Part model, mm, in its own coordinate system. Face numbers are marked on the shaded views. Coordinates: 2 decimals unless noted, no trailing zeros. Write each loop counter-clockwise with the first axis right and the second up, starting at its lowest first coordinate (ties: lowest second). Pieces come first, ordered by that corner, then holes. Notation, with made-up numbers: (1.25, 29.25) - (20.25, 29.25) arc R20 cw to (20.25, 57.25) - close; hole circle Ø10 at (-20, 2). An arc over 180 degrees is marked (long way). Use a Markdown table: item, result.
```python
from build123d import *

# Parameters (mm, degrees)
STOCK_MULTIBODY_1_OUTLINE_R   = 1.6
STOCK_MULTIBODY_1_OUTLINE_R_2 = 8.85
STOCK_MULTIBODY_1_DEPTH       = 17.5
CUT_EXTRUDE1_DEPTH            = 33.06633749
CUT_EXTRUDE1_DEPTH_BACK       = 33.06633749
SKETCH1_R                     = 17.5


# Read off the part's stored shape, not the designer's step: Stock-Multibody-1
with BuildPart() as part:
    # Stock-Multibody-1 outline → Stock-Multibody-1 (new body)
    with BuildSketch(Plane(origin=(0, 0, 0), x_dir=(1, 0, 0), z_dir=(0, 1, 0))):
        with BuildLine():
            ThreePointArc((-19, -17), (-18.414213562, -18.414213562), (-17, -19))
            Line((-17, -19), (17, -19))
            ThreePointArc((17, -19), (18.414213562, -18.414213562), (19, -17))
            Line((19, -17), (19, 17))
            ThreePointArc((19, 17), (18.414213562, 18.414213562), (17, 19))
            Line((17, 19), (-17, 19))
            ThreePointArc((-17, 19), (-18.414213562, 18.414213562), (-19, 17))
            Line((-19, 17), (-19, -17))
        make_face()
        with Locations((-14.8, -14.8)):
            Circle(STOCK_MULTIBODY_1_OUTLINE_R, mode=Mode.SUBTRACT)
        with Locations((14.8, -14.8)):
            Circle(STOCK_MULTIBODY_1_OUTLINE_R, mode=Mode.SUBTRACT)
        with Locations((-14.8, 14.8)):
            Circle(STOCK_MULTIBODY_1_OUTLINE_R, mode=Mode.SUBTRACT)
        Circle(STOCK_MULTIBODY_1_OUTLINE_R_2, mode=Mode.SUBTRACT)
        with Locations((14.8, 14.8)):
            Circle(STOCK_MULTIBODY_1_OUTLINE_R, mode=Mode.SUBTRACT)
    extrude(amount=STOCK_MULTIBODY_1_DEPTH)

    # Sketch1 → Cut-Extrude1 (cut, two sides: drawn at the far end of the back side and taken through both)
    with BuildSketch(Plane(origin=(0, 17.5, 0), x_dir=(1, 0, 0), z_dir=(0, 1, 0)).offset(-CUT_EXTRUDE1_DEPTH_BACK)):
        with Locations(Location((0, 0, 0), (0, 0, 270))):
            Circle(SKETCH1_R)
    extrude(amount=CUT_EXTRUDE1_DEPTH + CUT_EXTRUDE1_DEPTH_BACK, mode=Mode.SUBTRACT)


solid = part.part
```
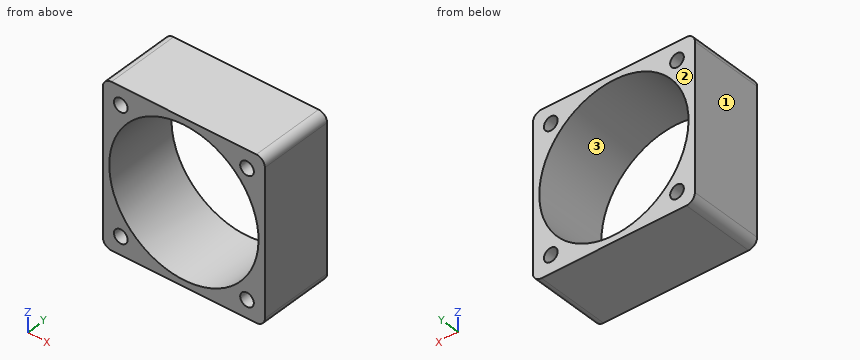
Item 1: Band-saw the part on C-C, the plane y = 9. Give the cut face in (x, z), then the cut area to 3 significant figures.
From the geometry:
| item | result |
|---|---|
| outline | (-19, -17) arc R2 ccw to (-17, -19) - (17, -19) arc R2 ccw to (19, -17) - (19, 17) arc R2 ccw to (17, 19) - (-17, 19) arc R2 ccw to (-19, 17) - close; hole circle Ø35 at (0, 0); hole circle Ø3.2 at (-14.8, -14.8); hole circle Ø3.2 at (-14.8, 14.8); hole circle Ø3.2 at (14.8, -14.8); hole circle Ø3.2 at (14.8, 14.8) |
| area | 446 mm^2 |
Item 2: Two-plate mould, pull along X, no slides. Class the marked faces 1, 2 and 3: pulls with the +X half, pulls with the -X half, needs draft (parallel to the pull), parting line crosses it, or undercut.
From the geometry:
| item | result |
|---|---|
| face 1 | pulls with the -X half |
| face 2 | needs draft |
| face 3 | undercut |
Item 3: Band-saw the part on D-D, the plane x = -15.5. Give the cut face in (y, z), then the cut area to 3 significant figures.
From the geometry:
| item | result |
|---|---|
| outline | (0, -19) - (17.5, -19) - (17.5, -16.24) - (0, -16.24) - close; (0, -13.36) - (17.5, -13.36) - (17.5, -8.12) - (0, -8.12) - close; (0, 8.12) - (17.5, 8.12) - (17.5, 13.36) - (0, 13.36) - close; (0, 16.24) - (17.5, 16.24) - (17.5, 19) - (0, 19) - close |
| area | 280 mm^2 |
Item 4: Band-saw the part on B-B, the plane z = 0. Give the cut face in (x, y), then the cut area to 3 significant figures.
From the geometry:
| item | result |
|---|---|
| outline | (-19, 0) - (-17.5, 0) - (-17.5, 17.5) - (-19, 17.5) - close; (17.5, 0) - (19, 0) - (19, 17.5) - (17.5, 17.5) - close |
| area | 52.5 mm^2 |
Item 5: Drill centre lines: probe 1 along Z at (x, y) = (0, 13.5); probe 2 along Z at (x, y) = (-14.8, 9). Where is each one in solid material? Low to high.
From the geometry:
| item | result |
|---|---|
| probe 1 | -19 to -17.5, 17.5 to 19 |
| probe 2 | -19 to -16.4, -13.2 to -9.34, 9.34 to 13.2, 16.4 to 19 |
Item 6: Band-saw the part on A-A, the plane x = 0. Give the cut face in (y, z), then the cut area to 3 significant figures.
From the geometry:
| item | result |
|---|---|
| outline | (0, -19) - (17.5, -19) - (17.5, -17.5) - (0, -17.5) - close; (0, 17.5) - (17.5, 17.5) - (17.5, 19) - (0, 19) - close |
| area | 52.5 mm^2 |
